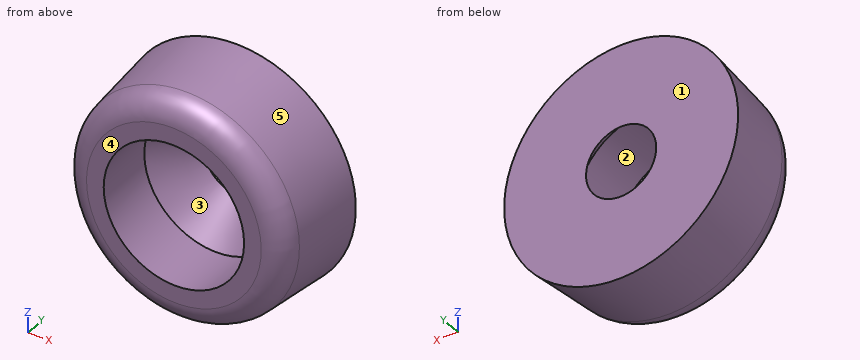
```python
from build123d import *

# Parameters (mm, degrees)
SKETCH_1_R          = 5
EXTRUDE_1_DEPTH     = 4
SKETCH_2_R          = 1.5
CUT_EXTRUDE_1_DEPTH = 5
DRAFT_1_ANGLE       = -1
DRAFT_4_ANGLE       = -5
SKETCH_3_R          = 3
CUT_EXTRUDE_2_DEPTH = 2
FILLET_1_R          = 1
CHAMFER_1_SIZE      = 2


with BuildPart() as part:
    # Эскиз1 → Бобышка-Вытянуть1 (new body)
    with BuildSketch(Plane(origin=(0, 0, 0), x_dir=(1, 0, 0), z_dir=(0, 1, 0))):
        with Locations(Location((0, 0, 0), (0, 0, 270))):
            Circle(SKETCH_1_R)
    extrude(amount=EXTRUDE_1_DEPTH)

    # Эскиз2 → Вырез-Вытянуть1 (cut)
    with BuildSketch(Plane(origin=(0, 4, 0), x_dir=(1, 0, 0), z_dir=(0, 1, 0))):
        with Locations(Location((0, 0, 0), (0, 0, 270))):
            Circle(SKETCH_2_R)
    extrude(amount=-CUT_EXTRUDE_1_DEPTH, mode=Mode.SUBTRACT)

    # Уклон1
    draft_1_faces = [part.faces().sort_by_distance(p)[0] for p in [
        (0, 2, -5),
    ]]
    draft(draft_1_faces, Plane.ZX.offset(4), DRAFT_1_ANGLE)

    # Уклон4
    draft_4_faces = [part.faces().sort_by_distance(p)[0] for p in [
        (0, 2, -4.96508987),
    ]]
    draft(draft_4_faces, Plane.ZX.offset(4), DRAFT_4_ANGLE)

    # Эскиз3 → Вырез-Вытянуть2 (cut)
    with BuildSketch(Plane.XZ):
        with Locations(Location((0, 0, 0), (0, 0, 270))):
            Circle(SKETCH_3_R)
    extrude(amount=-CUT_EXTRUDE_2_DEPTH, mode=Mode.SUBTRACT)

    # Скругление1
    fillet_1_edges = [part.edges().sort_by_distance(p)[0] for p in [
        (0, 0, -4.650045346),
    ]]
    fillet(fillet_1_edges, radius=FILLET_1_R)

    # Фаска1
    # the kernel refuses this chamfer: 2 mm, written as the material it takes off along each edge
    with BuildSketch(Plane(origin=(0, 2, 0), x_dir=(0, 0, 1), z_dir=(-1, 0, 0))) as chamfer_1_piece_1_section:
        Polygon((1.5, CHAMFER_1_SIZE), (1.5 + CHAMFER_1_SIZE, 0), (1.5, 0), align=None)
    chamfer_1_piece_1 = revolve(axis=Axis((0, 2, 0), (0, 1, 0)), mode=Mode.PRIVATE)
    chamfer_1_piece_1 = chamfer_1_piece_1 & Plane(origin=(0, 3.257194568, 0), x_dir=(0, 0, -1), z_dir=(0, -1, 0)) * Cylinder(3, 14, mode=Mode.PRIVATE)
    add(chamfer_1_piece_1, mode=Mode.SUBTRACT)


solid = part.part
```
Read the model definition and answer for the solid it produces. Units are mm, in the model's axes. Face numbers are marked on the shaded views. A direction names the side the tool comes from. Coordinates: 2 decimals unless noted, no trailing zeros. Write each loop counter-clockwise with the first axis right and the second up, starting at its lowest first coordinate (ties: lowest second). Pieces come first, ordered by that corner, then holes. Notation, with made-up numbers: (71, 53) - (77, 53) arc R21 ccw to (77, 58) - close; hole circle Ø2 at (32.5, 24.5). An arc over 180 degrees is marked (long way). Answer as a JSON object with one key per item and string values. Group by question number.
1. A cutting plane is placed at B-B (z = 0). Determine the outline of the cut face in (x, y).
2. Which of the six approach directions +Z, -Z, +X, -X, +Y, -Y give full straight-line access (tool end or side, diameter ignored) to the marked faces 1 and 2?
3. Each of these flat-tipped pins is pushed along its axis until it touches: P1, Ø2, axis at y = 2, z = 0, coming from the -X side; P2, Ø1.5, axis at x = -3.5, y = 3, coming from the +Z side; P3, Ø2, axis at x = 2, y = 3.5, coming from the -Z side. Where does it stop, or does it pass through?
4. A cutting plane is placed at C-C (y = 2.95). Determine the outline of the cut face in (x, z), plus the area to 3 significant figures.
5. A cutting plane is placed at D-D (y = 1.85). Determine the outline of the cut face in (x, z).
6. The mould has two halves that part along Z. Classify the marked faces 3, 4 and 5: +Z half, -Z half, draft (parallel to the pull), parting line (faces both ways), or undercut.
7. Consider L1, parallel to Z at x = -2.25, y = 2.15; L2, parallel to X at y = 0.9, z = 0; L3, parallel to Z at x = 0, y = 1.6. Determine where each line is inside the solid, lowest interval first. Write a range as [from, to].
8. A cutting plane is placed at A-A (x = 0). Determine the outline of the cut face in (y, z).
Worked out:
{
 "1": {"outline": "(-5, 4) - (-4.73, 0.91) arc R1 ccw to (-3.73, 0) - (-3, 0) - (-3, 2.5) - (-1.5, 4) - close; (1.5, 4) - (3, 2.5) - (3, 0) - (3.73, 0) arc R1 ccw to (4.73, 0.91) - (5, 4) - close"},
 "2": {"face 1": "+Z, -Z, +X, -X, +Y", "face 2": "-Y"},
 "3": {"P1": "stops at x = -4.91", "P2": "stops at z = 4.08", "P3": "stops at z = -4.87"},
 "4": {"outline": "circle Ø9.82 at (0, 0); hole circle Ø5.1 at (0, 0)", "area": "55.3 mm²"},
 "5": {"outline": "circle Ø9.62 at (0, 0); hole circle Ø6 at (0, 0)"},
 "6": {"face 3": "undercut", "face 4": "draft", "face 5": "parting line"},
 "7": {"L1": "z = [-4.28, -1.98], [1.98, 4.28]", "L2": "x = [-4.73, -3], [3, 4.73]", "L3": "z = [-4.79, -3], [3, 4.79]"},
 "8": {"outline": "(0, -3.73) arc R1 ccw to (0.91, -4.73) - (4, -5) - (4, -1.5) - (2.5, -3) - (0, -3) - close; (0, 3) - (2.5, 3) - (4, 1.5) - (4, 5) - (0.91, 4.73) arc R1 ccw to (0, 3.73) - close"}
}
